Model file for the job. Use its own axes, mm. Coordinates: 2 decimals unless noted, no trailing zeros. Order: outer loops, then holes, each group sorted by start corner. A loop starts at its lowest first (then second) coordinate and runs counter-clockwise, first axis right, second up. Notation, with made-up numbers: M 19.5,-9.75 L 32.5,-9.75 A37 cw 32.5,28.25 Z; hole C 52.5,-35 d8. An arc over 180 degrees is marked long. Return JSON: item names as keys, results as strings.
```python
from build123d import *

# Parameters (mm, degrees)
SKETCH1_R           = 1.75
BOSS_EXTRUDE1_DEPTH = 2.5
FILLET1_R           = 10


with BuildPart() as part:
    # Sketch1 → Boss-Extrude1 (new body)
    with BuildSketch(Plane.XY):
        with BuildLine():
            ThreePointArc((-23.625, 3.25), (-26.875, 0), (-23.625, -3.25))
            Line((-23.625, -3.25), (0, -7.5))
            Line((0, -7.5), (23.625, -3.25))
            ThreePointArc((23.625, -3.25), (26.875, 0), (23.625, 3.25))
            Line((23.625, 3.25), (0, 7.5))
            Line((0, 7.5), (-23.625, 3.25))
        make_face()
        with Locations((-23.625, 0)):
            Circle(SKETCH1_R, mode=Mode.SUBTRACT)
        Circle(SKETCH1_R, mode=Mode.SUBTRACT)
        with Locations((23.625, 0)):
            Circle(SKETCH1_R, mode=Mode.SUBTRACT)
    extrude(amount=BOSS_EXTRUDE1_DEPTH)

    # Fillet1
    fillet1_edges = [part.edges().sort_by_distance(p)[0] for p in [
        (0, -7.5, 1.25),
        (0, 7.5, 1.25),
    ]]
    fillet(fillet1_edges, radius=FILLET1_R)


solid = part.part
```
Item 1: Saw through at C-C (z = 0.95). Count the separate pieces of the cut face and the enclosed holes in it, and give its area (3 significant figures).
Check result:
{"separate pieces": "1", "enclosed holes": "3", "area": "512 mm2"}
Item 2: Saw through at B-B (x = 0). Write the cut outline in (y, z).
Check result:
{"outline": "M -7.34,0 L -1.75,0 L -1.75,2.5 L -7.34,2.5 Z; M 1.75,0 L 7.34,0 L 7.34,2.5 L 1.75,2.5 Z"}
Item 3: Pull direction X, two halves, no side cores. Call faces 1 (the cylindrical face through (-0.02, -7.34, 1.27)), 2 (the flat face through (-12.85, -5.19, 1.23)), 3 (the cylindrical face through (1.617, -0.67, 1.232)): +X half, -X half, draft (parallel to the pull), parting line (faces both ways), or undercut.
Check result:
{"face 1": "parting line", "face 2": "-X half", "face 3": "undercut"}
Item 4: Saw through at A-A (y = 0). Write the cut outline in (x, z) (3 decimals), and give its area (3 significant figures).
Check result:
{"outline": "M -26.875,0 L -25.375,0 L -25.375,2.5 L -26.875,2.5 Z; M -21.875,0 L -1.75,0 L -1.75,2.5 L -21.875,2.5 Z; M 1.75,0 L 21.875,0 L 21.875,2.5 L 1.75,2.5 Z; M 25.375,0 L 26.875,0 L 26.875,2.5 L 25.375,2.5 Z", "area": "108 mm2"}
Item 5: Wall check: line 1 (X direction, y = -1.25, z = 0.5) (3 decimals); line 2 (X direction, y = 0.25, z = 1.4); line 3 (Y direction, x = 12, z = 1.75). Give the ranges that are in metal, low to high.
Check result:
{"line 1": "x = -26.625 to -24.85, -22.4 to -1.225, 1.225 to 22.4, 24.85 to 26.625", "line 2": "x = -26.87 to -25.36, -21.89 to -1.73, 1.73 to 21.89, 25.36 to 26.87", "line 3": "y = -5.34 to 5.34"}
Item 6: Saw through at D-D (x = -22.5). Write the cut outline in (y, z), and give its area (3 significant figures).
Check result:
{"outline": "M -3.45,0 L -1.34,0 L -1.34,2.5 L -3.45,2.5 Z; M 1.34,0 L 3.45,0 L 3.45,2.5 L 1.34,2.5 Z", "area": "10.6 mm2"}
